```python
from build123d import *

# Parameters (mm, degrees)
CYLINDER_R       = 2
CYLINDER_DEPTH   = 100
ARRAY002_X_COUNT = 2
ARRAY002_X_PITCH = 77
BOX009_W         = 30
BOX009_H         = 10
BOX009_DEPTH     = 14.5
BOX001_W         = 142.4
BOX001_H         = 71
BOX001_DEPTH     = 13.3
BOX_W            = 146.4
BOX_H            = 74
BOX_DEPTH        = 12.8
FILLET_R         = 1.5


with BuildPart() as obj1:
    # Cylinder → Cylinder (new body)
    with BuildSketch(Plane(origin=(9.5, -16, 3.5), x_dir=(1, 0, 0), z_dir=(0, 1, 0))):
        Circle(CYLINDER_R)
    extrude(amount=CYLINDER_DEPTH)

    # Array002 X: obj1_2


with BuildPart() as obj1_1:
    add(obj1.part)
    with Locations(*[(i * ARRAY002_X_PITCH, 0, 0) for i in range(1, ARRAY002_X_COUNT)]):
        add(obj1.part)


with BuildPart() as obj1_2:
    # Body placement: moved
    add(obj1_1.part.moved(Location((2.2, 0, 2.9))))


with BuildPart() as usb_extent_hole:
    # Box009 → Box009 (new body)
    with BuildSketch(Plane(origin=(131, 27.5, 1.4), x_dir=(1, 0, 0), z_dir=(0, 0, 1))):
        with Locations((15, 5)):
            Rectangle(BOX009_W, BOX009_H)
    extrude(amount=BOX009_DEPTH)


with BuildPart() as bottom_body_hole_fusion:
    # Box001 → Box001 (new body)
    with BuildSketch(Plane(origin=(2, 1.5, 1), x_dir=(1, 0, 0), z_dir=(0, 0, 1))):
        with Locations((71.2, 35.5)):
            Rectangle(BOX001_W, BOX001_H)
    extrude(amount=BOX001_DEPTH)

    # Fusion: union obj1, usb extent hole
    add(obj1_2.part)
    add(usb_extent_hole.part)


with BuildPart() as bottom_fillet:
    # Box → Box (new body)
    with BuildSketch(Plane.XY):
        with Locations((73.2, 37)):
            Rectangle(BOX_W, BOX_H)
    extrude(amount=BOX_DEPTH)

    # Cut: cut bottom body hole fusion
    add(bottom_body_hole_fusion.part, mode=Mode.SUBTRACT)

    # Fillet
    fillet_edges = [bottom_fillet.edges().sort_by_distance(p)[0] for p in [
        (0, 0, 6.4),
        (0, 74, 6.4),
        (146.4, 0, 6.4),
        (146.4, 74, 6.4),
        (144.4, 72.5, 6.9),
        (144.4, 1.5, 6.9),
        (2, 72.5, 6.9),
        (2, 1.5, 6.9),
    ]]
    fillet(fillet_edges, radius=FILLET_R)


solid = bottom_fillet.part
```
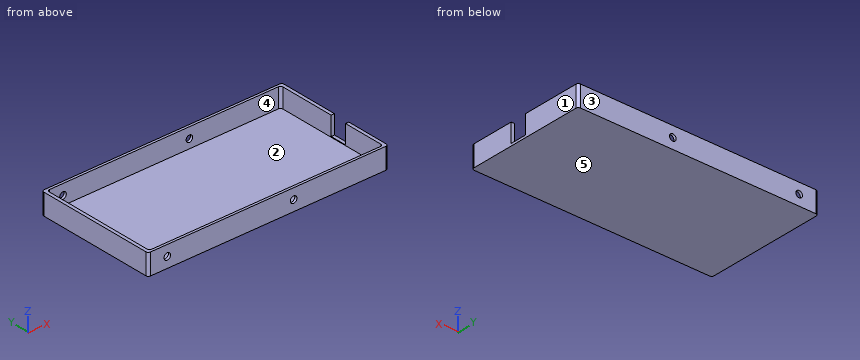
Geometry check sheet. Reference: the model listing, model coordinates, mm. Face numbers are marked on the shaded views. A direction names the side the tool comes from. Round coordinates to 2 decimals unless told otherwise and drop trailing zeros. Loops run counter-clockwise (first coordinate to the right, second up) from the corner with the lowest first, then second, coordinate; pieces in that order, holes last. Notation, with made-up numbers: (-23.5, 70) - (35.5, 70) arc R24 ccw to (35.5, 81) - close; hole circle Ø11 at (-29.5, 26). An arc over 180 degrees is marked (long way). Write item = value, one per line. Start each with the question number.
1. Depth check by flat-ended pin: pin 1 (0.6 mm diameter, centred on x = 145, y = 35, fed in from +Z); pin 2 (3 mm diameter, centred on x = 16.5, y = 28.5, fed in from +Z); pin 3 (0.6 mm diameter, centred on x = 145.5, z = 6.5, fed in from -Y). Enter the tip coordinate at first touch or a pass-through.
2. Section check B-B on x = 56. Enter the section's corners in (y, z), then the cut area to 3 significant figures.
3. Thickness scan on line 1 (Z direction, x = 88.7, y = 73); line 2 (X direction, y = 24, z = 6.25); line 3 (Y direction, x = 134, z = 5.25). Record the ranges inside material, lowest first.
4. Section check A-A on x = 88.7. Enter the section's corners in (y, z).
5. Mould release check, pull along Y, two halves, no side actions. Record for the marked faces 3, 4 and 5: released by +Y, released by -Y, zero draft, split by the parting line, or undercut.
6. Section check C-C on z = 10.5. Enter the section's corners in (x, y).
7. Set-up check for the marked faces 1 and 2: record each of +Z, -Z, +X, -X, +Y, -Y from which the full face is reachable in a straight line by a thin tool's end or side.
8. Section check D-D on y = 49. Enter the section's corners in (x, z).
Working result:
q1.pin_1 = 1.4
q1.pin_2 = 1
q1.pin_3 = 0.03
q2.outline = (0, 0) - (74, 0) - (74, 12.8) - (72.5, 12.8) - (72.5, 1) - (1.5, 1) - (1.5, 12.8) - (0, 12.8) - close
q2.area = 109 mm^2
q3.line_1 = 0 to 4.4, 8.4 to 12.8
q3.line_2 = 0 to 2, 144.4 to 146.4
q3.line_3 = 0 to 1.5, 72.5 to 74
q4.outline = (0, 0) - (74, 0) - (74, 4.4) - (72.5, 4.4) - (72.5, 1) - (1.5, 1) - (1.5, 4.4) - (0, 4.4) - close; (0, 8.4) - (1.5, 8.4) - (1.5, 12.8) - (0, 12.8) - close; (72.5, 8.4) - (74, 8.4) - (74, 12.8) - (72.5, 12.8) - close
q5.face_3 = released by +Y
q5.face_4 = undercut
q5.face_5 = zero draft
q6.outline = (0, 1.5) arc R1.5 ccw to (1.5, 0) - (144.9, 0) arc R1.5 ccw to (146.4, 1.5) - (146.4, 27.5) - (144.4, 27.5) - (144.4, 3) arc R1.5 cw to (142.9, 1.5) - (3.5, 1.5) arc R1.5 cw to (2, 3) - (2, 71) arc R1.5 cw to (3.5, 72.5) - (142.9, 72.5) arc R1.5 cw to (144.4, 71) - (144.4, 37.5) - (146.4, 37.5) - (146.4, 72.5) arc R1.5 ccw to (144.9, 74) - (1.5, 74) arc R1.5 ccw to (0, 72.5) - close
q7.face_1 = +Z, -Z, +X, +Y, -Y
q7.face_2 = +Z
q8.outline = (0, 0) - (146.4, 0) - (146.4, 12.8) - (144.4, 12.8) - (144.4, 1) - (2, 1) - (2, 12.8) - (0, 12.8) - close
